Here's how the part is built. I have some questions about the finished solid (model axes, mm). Face numbers are marked on the shaded views. A direction names the side the tool comes from. Round coordinates to 2 decimals unless told otherwise and drop trailing zeros. Order: outer loops, then holes, each group sorted by start corner. A loop starts at its lowest first (then second) coordinate and runs counter-clockwise, first axis right, second up.
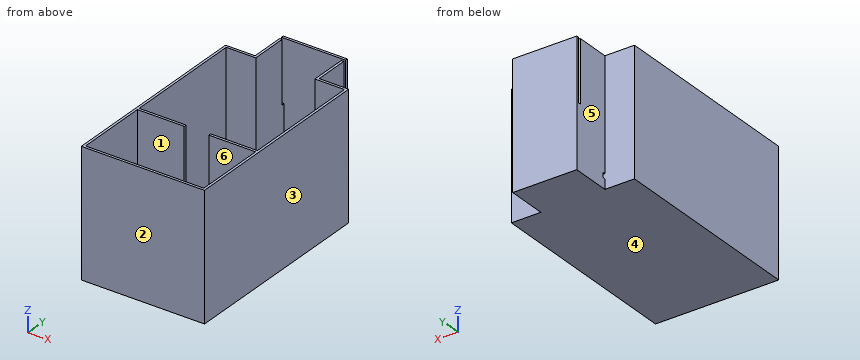
Autodesk Inventor part; units mm, degrees
ref_plane "YZ Plane" through (0, 0, 0) normal (1, 0, 0) x (0, 1, 0)
ref_plane "XZ Plane" through (0, 0, 0) normal (0, 1, 0) x (-1, 0, 0)
ref_plane "XY Plane" through (0, 0, 0) normal (0, 0, 1) x (1, 0, 0)
sketch "스케치1" plane through (0, 0, 0) normal (0, 0, 1) x (1, 0, 0)
  line L0 (0, 0) -> (500, 0)
  line L1 (500, 0) -> (500, 820)
  line L2 (0, 0) -> (0, 820)
  line L3 (0, 820) -> (120, 820)
  line L4 (120, 820) -> (120, 980)
  line L5 (120, 980) -> (380, 980)
  line L6 (380, 980) -> (380, 820)
  line L7 (380, 820) -> (500, 820)
  line L8 (10, 10) -> (490, 10)
  line L9 (490, 10) -> (490, 305)
  line L10 (490, 305) -> (300, 305)
  line L11 (300, 305) -> (300, 315)
  line L12 (300, 315) -> (490, 315)
  line L13 (490, 315) -> (490, 810)
  line L14 (490, 810) -> (370, 810)
  line L15 (370, 810) -> (370, 970)
  line L16 (370, 970) -> (130, 970)
  line L17 (130, 970) -> (130, 810)
  line L18 (130, 810) -> (10, 810)
  line L19 (10, 810) -> (10, 315)
  line L20 (10, 315) -> (200, 315)
  line L21 (200, 315) -> (200, 305)
  line L22 (200, 305) -> (10, 305)
  line L23 (10, 305) -> (10, 10)
  dimension "d0" = 500
  dimension "d1" = 820
  dimension "d2" = 820
  dimension "d3" = 10
  dimension "d4" = 10
  dimension "d5" = 10
  dimension "d6" = 10
  dimension "d7" = 10
  dimension "d8" = 10
  dimension "d9" = 10
  dimension "d10" = 10
  dimension "d11" = 100
  dimension "d12" = 295
  dimension "d13" = 240
  dimension "d14" = 160
extrude "돌출1" add sketch "스케치1" along normal blind 500
sketch "스케치2" plane through (0, 0, 0) normal (0, 0, -1) x (-1, 0, 0)
  line L0 (-380, 820) -> (-380, 980)
  line L1 (-500, 820) -> (-380, 820)
  line L2 (-500, 0) -> (-500, 820)
  line L3 (0, 0) -> (-500, 0)
  line L4 (0, 820) -> (0, 0)
  line L5 (-120, 820) -> (0, 820)
  line L6 (-120, 980) -> (-120, 820)
  line L7 (-380, 980) -> (-120, 980)
  line L8 (-490, 305) -> (-490, 10)
  line L9 (-300, 305) -> (-490, 305)
  line L10 (-300, 315) -> (-300, 305)
  line L11 (-490, 315) -> (-300, 315)
  line L12 (-490, 810) -> (-490, 315)
  line L13 (-370, 810) -> (-490, 810)
  line L14 (-370, 970) -> (-370, 810)
  line L15 (-130, 970) -> (-370, 970)
  line L16 (-130, 810) -> (-130, 970)
  line L17 (-10, 810) -> (-130, 810)
  line L18 (-10, 315) -> (-10, 810)
  line L19 (-200, 315) -> (-10, 315)
  line L20 (-200, 305) -> (-200, 315)
  line L21 (-10, 305) -> (-200, 305)
  line L22 (-10, 10) -> (-10, 305)
  line L23 (-490, 10) -> (-10, 10)
extrude "돌출2" add sketch "스케치2" along normal blind 10 contours L0 L7 L6 L5 L4 L3 L2 L1 | L9 L10 L11 L12 L13 L14 L15 L16 L17 L18 L19 L20 L21 L22 L23 L8
sketch "스케치3" plane through (0, 0, 500) normal (0, 0, 1) x (1, 0, 0)
  line L0 (380, 820) -> (380, 980)
  line L1 (380, 980) -> (120, 980)
  line L2 (120, 980) -> (120, 820)
  line L3 (120, 820) -> (0, 820)
  line L4 (0, 820) -> (0, 0)
  line L5 (0, 0) -> (500, 0)
  line L6 (500, 0) -> (500, 820)
  line L7 (500, 820) -> (380, 820)
  line L8 (490, 305) -> (490, 10)
  line L9 (490, 10) -> (10, 10)
  line L10 (10, 10) -> (10, 305)
  line L11 (10, 305) -> (200, 305)
  line L12 (200, 305) -> (200, 315)
  line L13 (200, 315) -> (10, 315)
  line L14 (10, 315) -> (10, 810)
  line L15 (10, 810) -> (130, 810)
  line L16 (130, 810) -> (130, 970)
  line L17 (130, 970) -> (370, 970)
  line L18 (370, 970) -> (370, 810)
  line L19 (370, 810) -> (490, 810)
  line L20 (490, 810) -> (490, 315)
  line L21 (490, 315) -> (300, 315)
  line L22 (300, 315) -> (300, 305)
  line L23 (300, 305) -> (490, 305)
  line L24 (120, 980) -> (120, 820)
  line L25 (380, 820) -> (380, 980)
  line L26 (120, 960) -> (380, 960)
  line L27 (380, 960) -> (380, 970)
  line L28 (380, 970) -> (120, 970)
  line L29 (120, 970) -> (120, 960)
  line L30 (130, 970) -> (370, 970)
  point P0 (370, 960)
  point P1 (130, 960)
  dimension "d19" = 10
extrude "돌출3" cut sketch "스케치3" against normal blind 250 contours L26 L18 L28 L0 | L26 L2 L28 L16
sketch "스케치4" plane through (380, 820, -10) normal (1, 0, 0) x (0, 0, -1)
  line L0 (0, 160) -> (0, 0)
  line L1 (0, 0) -> (-510, 0)
  line L2 (-40, 0) -> (-60, 0)
  line L3 (-60, 0) -> (-60, 10)
  line L4 (-60, 10) -> (-40, 10)
  line L5 (-40, 10) -> (-40, 0)
  line L6 (-10, -505) -> (-10, -10)
  point P0 (-10, -820)
  dimension "d22" = 20
  dimension "d23" = 10
  dimension "d24" = 30
extrude "돌출4" cut sketch "스케치4" against normal through all
properties part number "Main"
1) I'm going to push a flat-ended pin straight in: pin 1 (5 mm diameter, centred on x = 241.5, y = 395, fed in from +Z). Where does the tip first touch, or does it pass through?
2) If we section it at B-B (x = 210.5): Write out the boundary of the cut face in (y, z).
3) If we section it at D-D (z = 198): Write out the boundary of the cut face in (x, y), plus the area to 3 significant figures.
4) For the marked faces 4, 5 and 6, which set-ups out of +Z, -Z, +X, -X, +Y, -Y let a thin tool reach every point of the face, with its end or its side?
5) If we section it at A-A (z = 349): Write out the boundary of the cut face in (x, y), plus the area to 3 significant figures.
6) We'd pull the mould along X, two halves only. Please class the marked faces 1, 2 and 3: +X half, -X half, draft (parallel to the pull), parting line (faces both ways), or undercut.
7) If we section it at C-C (y = 707.5): Write out the boundary of the cut face in (x, z), plus the area to 3 significant figures.
8) I need wall thicknesses on line 1 (Y direction, x = 468, z = 330); line 2 (Y direction, x = 303.5, z = 79); line 3 (X direction, y = 567.5, z = 338). Which ranges of each line are inside material? Lowest first, please.
Solutions:
1. pin 1: stops at z = 0
2. outline: (0, -10) - (980, -10) - (980, 500) - (970, 500) - (970, 0) - (10, 0) - (10, 500) - (0, 500) - close
3. outline: (0, 0) - (500, 0) - (500, 820) - (380, 820) - (380, 980) - (120, 980) - (120, 820) - (0, 820) - close; hole (10, 10) - (490, 10) - (490, 305) - (300, 305) - (300, 315) - (490, 315) - (490, 810) - (370, 810) - (370, 970) - (130, 970) - (130, 810) - (10, 810) - (10, 315) - (200, 315) - (200, 305) - (10, 305) - close
3. area: 33,000 mm2
4. face 4: -Z, +X, -X, +Y, -Y
4. face 5: +Z, -Z, -X, +Y
4. face 6: +Z
5. outline: (0, 0) - (500, 0) - (500, 820) - (380, 820) - (380, 960) - (370, 960) - (370, 810) - (490, 810) - (490, 315) - (300, 315) - (300, 305) - (490, 305) - (490, 10) - (10, 10) - (10, 305) - (200, 305) - (200, 315) - (10, 315) - (10, 810) - (130, 810) - (130, 960) - (120, 960) - (120, 820) - (0, 820) - close; (120, 970) - (380, 970) - (380, 980) - (120, 980) - close
5. area: 32,800 mm2
6. face 1: undercut
6. face 2: draft
6. face 3: +X half
7. outline: (0, -10) - (500, -10) - (500, 500) - (490, 500) - (490, 0) - (10, 0) - (10, 500) - (0, 500) - close
7. area: 15,000 mm2
8. line 1: y = 0 to 10, 305 to 315, 810 to 820
8. line 2: y = 0 to 10, 305 to 315, 970 to 980
8. line 3: x = 0 to 10, 490 to 500
